Verification items for the finished model (mm, model axes). Coordinates: 2 decimals unless noted, no trailing zeros. Order: outer loops, then holes, each group sorted by start corner. A loop starts at its lowest first (then second) coordinate and runs counter-clockwise, first axis right, second up. Notation, with made-up numbers: (3, -37) -> (7, -37) arc R21 ccw to (7, -22) -> close; hole circle Ø7 at (83.25, 86.5). An arc over 180 degrees is marked (long way). Use CSV: the item, a comma, the result in double quotes. Start each with the question number.
1) Sectioned sample at C-C on x = 52.5. Record the boundary of the cut face in (y, z) (3 decimals), then the cut area to 3 significant figures.
2) Sectioned sample at B-B on z = 1.3. Give the number of separate pieces and of enclosed holes in the cut face, then the cut area to 3 significant figures.
3) Go/stop test with flat-tipped pins: pin 1 (1 mm diameter, centred on x = 16.5, z = 1.5, fed in from -Y) (3 decimals); pin 2 (2 mm diameter, centred on x = -46.55, y = -46.36, fed in from -Z) (3 decimals). Record where each tip stops, or that it passes through.
4) Scan lines: line 1 along Y through (x, z) = (88.9, 2) (3 decimals); line 2 along Y through (x, z) = (-96.02, 2.3) (3 decimals); line 3 along Y through (x, z) = (-67, 2.4) (3 decimals). Record each from-to range of solid material in increasing order.
5) Sectioned sample at A-A on x = -69.5. Record the boundary of the cut face in (y, z) (3 decimals), then the cut area to 3 significant figures.
from build123d import *

# Parameters (mm, degrees)
F0_R     = 1.85
F0_R_2   = 2.35
F0_W     = 40.9
F0_H     = 19.9
F1_DEPTH = 3


with BuildPart() as f1:
    # F0 (on Top) → F1 (new body)
    with BuildSketch(Plane.XY):
        with BuildLine():
            Line((-152.4, 47.625), (-152.4, -47.625))
            Line((-152.4, -47.625), (-117.734805, -47.625))
            ThreePointArc((-117.734805, -47.625), (-116.932919, -47.610153), (-116.131032, -47.625))
            ThreePointArc((-116.131032, -47.625), (-107.434809, -49.803392), (-100.365224, -55.316166))
            ThreePointArc((-100.365224, -55.316166), (-98.186821, -56.982665), (-95.5088, -57.575))
            Line((-95.5088, -57.575), (-77.11, -57.575))
            Line((-77.11, -57.575), (-49.415637, -57.575))
            ThreePointArc((-49.415637, -57.575), (-46.989367, -57.093195), (-44.931282, -55.720894))
            ThreePointArc((-44.931282, -55.720894), (-36.753686, -50.062559), (-27.112724, -47.625))
            Line((-27.112724, -47.625), (152.4, -47.625))
            Line((152.4, -47.625), (152.4, 47.625))
            Line((152.4, 47.625), (-152.4, 47.625))
        make_face()
        with Locations((-96.02, -46.36)):
            Circle(F0_R, mode=Mode.SUBTRACT)
        with Locations((-139.7, -34.925)):
            Circle(F0_R_2, mode=Mode.SUBTRACT)
        with Locations((-96.02, -36.19)):
            Circle(F0_R, mode=Mode.SUBTRACT)
        with Locations((-46.55, -46.36)):
            Circle(F0_R, mode=Mode.SUBTRACT)
        with Locations((-71.8, -41.275)):
            Rectangle(F0_W, F0_H, mode=Mode.SUBTRACT)
        with Locations((-46.55, -36.19)):
            Circle(F0_R, mode=Mode.SUBTRACT)
        with Locations((31.75, -41.275)):
            Circle(F0_R_2, mode=Mode.SUBTRACT)
        with Locations((88.9, -34.925)):
            Circle(F0_R_2, mode=Mode.SUBTRACT)
    extrude(amount=F1_DEPTH)


solid = f1.part
Answers follow:
1,outline,"(-47.625, 0) -> (47.625, 0) -> (47.625, 3) -> (-47.625, 3) -> close"
1,area,"286 mm²"
2,separate pieces,"1"
2,enclosed holes,"8"
2,area,"28,800 mm²"
3,pin 1,"stops at y = -47.625"
3,pin 2,"passes through"
4,line 1,"y = -47.625 to -37.275, -32.575 to 47.625"
4,line 2,"y = -57.554 to -48.21, -44.51 to -38.04, -34.34 to 47.625"
4,line 3,"y = -57.575 to -51.225, -31.325 to 47.625"
5,outline,"(-57.575, 0) -> (-51.225, 0) -> (-51.225, 3) -> (-57.575, 3) -> close; (-31.325, 0) -> (47.625, 0) -> (47.625, 3) -> (-31.325, 3) -> close"
5,area,"256 mm²"
